from build123d import *

# Parameters (mm, degrees)
BOSS_EXTRUDE1_DEPTH = 3.175
SKETCH2_R           = 2.4892
CUT_EXTRUDE1_DEPTH  = 152.971856141
FILLET1_R           = 3.175


with BuildPart() as part:
    # Sketch1 → Boss-Extrude1 (new body)
    with BuildSketch(Plane.XY):
        Polygon((7.627179371, 56.026836403), (102.877179371, 5.226836403), (128.277179371, 5.226836403), (128.277179371, 81.426836403), (7.627179371, 81.426836403), align=None)
        Polygon((34.614679371, 56.026836403), (102.877179371, 56.026836403), (102.877179371, 19.620169736), align=None, mode=Mode.SUBTRACT)
    extrude(amount=BOSS_EXTRUDE1_DEPTH)

    # Sketch2 → Cut-Extrude1 (cut, through all)
    with BuildSketch(Plane.XY.offset(3.175)):
        with Locations((115.577179371, 43.326836403)):
            Circle(SKETCH2_R)
        with Locations((115.577179371, 17.926836403)):
            Circle(SKETCH2_R)
        with Locations((90.177179371, 68.726836403)):
            Circle(SKETCH2_R)
        with Locations((20.327179371, 68.726836403)):
            Circle(SKETCH2_R)
    extrude(amount=-CUT_EXTRUDE1_DEPTH, mode=Mode.SUBTRACT)

    # Fillet1
    fillet1_edges = [part.edges().sort_by_distance(p)[0] for p in [
        (34.614679371, 56.026836403, 1.5875),
        (102.877179371, 19.620169736, 1.5875),
        (102.877179371, 56.026836403, 1.5875),
        (128.277179371, 5.226836403, 1.5875),
        (102.877179371, 5.226836403, 1.5875),
        (7.627179371, 56.026836403, 1.5875),
        (7.627179371, 81.426836403, 1.5875),
        (128.277179371, 81.426836403, 1.5875),
    ]]
    fillet(fillet1_edges, radius=FILLET1_R)


solid = part.part
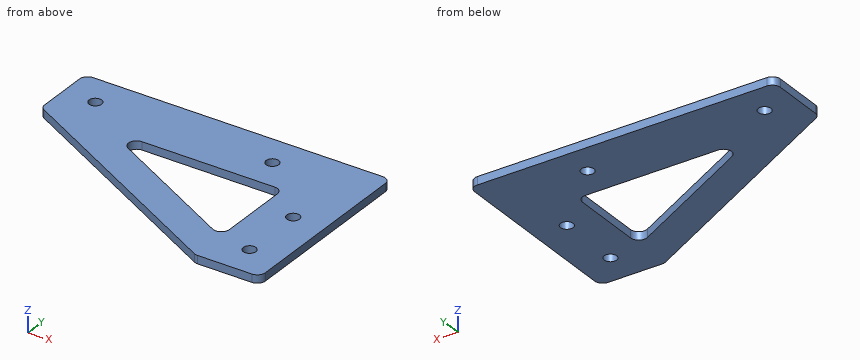
Read the model definition and answer for the solid it produces. Units are mm, in the model's axes. Round coordinates to 2 decimals unless told otherwise and drop trailing zeros. Write each loop counter-clockwise with the first axis right and the second up, starting at its lowest first coordinate (ties: lowest second). Pieces come first, ordered by that corner, then holes. Notation, with made-up numbers: M 25.25,0 L 71.25,0 A31 ccw 71.25,33 Z; hole C 27.5,9.25 d4. An arc over 180 degrees is marked long. Use a Markdown table: item, result.
1) The part is cut by section C-C (z = 1.2). Write down the section's boundary in (x, y) (3 decimals), plus the area to 3 significant figures.
Answers follow:
| item | result |
|---|---|
| outline | M 7.627,57.932 A3.175 ccw 9.308,55.13 L 102.177,5.6 A3.175 ccw 103.671,5.227 L 125.102,5.227 A3.175 ccw 128.277,8.402 L 128.277,78.252 A3.175 ccw 125.102,81.427 L 10.802,81.427 A3.175 ccw 7.627,78.252 Z; hole C 20.327,68.727 d4.978; hole M 45.821,50.05 L 98.208,22.11 A3.175 ccw 102.877,24.912 L 102.877,52.852 A3.175 ccw 99.702,56.027 L 47.315,56.027 A3.175 ccw Z; hole C 90.177,68.727 d4.978; hole C 115.577,17.927 d4.978; hole C 115.577,43.327 d4.978 |
| area | 5,480 mm2 |
2) The part is cut by section D-D (y = 32). Write down the section's boundary in (x, z) (1 decimal).
Answers follow:
| item | result |
|---|---|
| outline | M 52.7,0 L 79.7,0 L 79.7,3.2 L 52.7,3.2 Z; M 102.9,0 L 128.3,0 L 128.3,3.2 L 102.9,3.2 Z |
3) Straight lines are drawn through the part: line 1 along X through (y, z) = (42, 2) (1 decimal); line 2 along X through (y, z) = (30, 2.2) (1 decimal); line 3 along Y through (x, z) = (89.5, 1.7). For each, find the intervals that lie inside material, in ascending order. Write a range as [from, to].
Answers follow:
| item | result |
|---|---|
| line 1 | x = [33.9, 60.9], [102.9, 113.5], [117.7, 128.3] |
| line 2 | x = [56.4, 83.4], [102.9, 128.3] |
| line 3 | y = [12.36, 26.75], [56.03, 66.33], [71.12, 81.43] |
4) The part is cut by section A-A (x = 97). Write down the section's boundary in (y, z) (3 decimals).
Answers follow:
| item | result |
|---|---|
| outline | M 8.361,0 L 22.755,0 L 22.755,3.175 L 8.361,3.175 Z; M 56.027,0 L 81.427,0 L 81.427,3.175 L 56.027,3.175 Z |
5) The part is cut by section B-B (y = 70). Write down the section's boundary in (x, z) (3 decimals).
Answers follow:
| item | result |
|---|---|
| outline | M 7.627,0 L 18.188,0 L 18.188,3.175 L 7.627,3.175 Z; M 22.466,0 L 88.038,0 L 88.038,3.175 L 22.466,3.175 Z; M 92.316,0 L 128.277,0 L 128.277,3.175 L 92.316,3.175 Z |
6) A flat-ended cylindrical pin translates along its axis: pin 1 (4 mm diameter, centred on x = 115.58, y = 17.93, fed in from -Z). Find the tip coordinate at first contact, or state that the pin passes through.
Answers follow:
| item | result |
|---|---|
| pin 1 | passes through |
